Model file for the job. Use its own axes, mm. Face numbers are marked on the shaded views. A direction names the side the tool comes from. Coordinates: 2 decimals unless noted, no trailing zeros. Write each loop counter-clockwise with the first axis right and the second up, starting at its lowest first coordinate (ties: lowest second). Pieces come first, ordered by that corner, then holes. Notation, with made-up numbers: (47.5, 43.5) - (84.5, 43.5) arc R32 ccw to (84.5, 76.5) - close; hole circle Ø4 at (-9, -9.5). An arc over 180 degrees is marked (long way). Put each result on its own line as item: value. Start each with the question number.
1. Saw through at B-B, the plane z = -11. Write the cut outline in (x, y), plus the area to 3 significant figures.
2. Saw through at C-C, the plane x = -28. Write the cut outline in (y, z), plus the area to 3 significant figures.
3. Saw through at A-A, the plane y = -27.5. Write the cut outline in (x, z), plus the area to 3 significant figures.
4. Drop flat-ended pins along their axis: P1, Ø1.5, axis at x = -38, y = -27, coming from the -Z side; P2, Ø1, axis at x = -34, z = 12, coming from the -Y side; P3, Ø3, axis at x = -24, z = 1.5, coming from the +Y side; P4, Ø1.5, axis at x = -39.5, y = -28, coming from the +Z side. Give the stop position or say it passes through.
5. Pull direction Z, two halves, no side cores. Call the marked faces 1, 2, 3 and 4: released by +Z, released by -Z, zero draft, split by the parting line, or undercut.
6. Which spindle directions (+Z, -Z, +X, -X, +Y, -Y) get a long thin tool onto all of the face, cutting with end or side? Do the marked faces 5, 6 and 7. Say none if no direction does.
7. Saw through at D-D, the plane y = -9.75. Write the cut outline in (x, z), plus the area to 3 significant figures.
8. Drill centre lines: L1, parallel to Z at x = -40, y = -27.5; L2, parallel to Z at x = -36, y = -12.5; L3, parallel to Y at x = -34, z = -6. Where is each one in solid material? Low to high. Write a range as from..to.
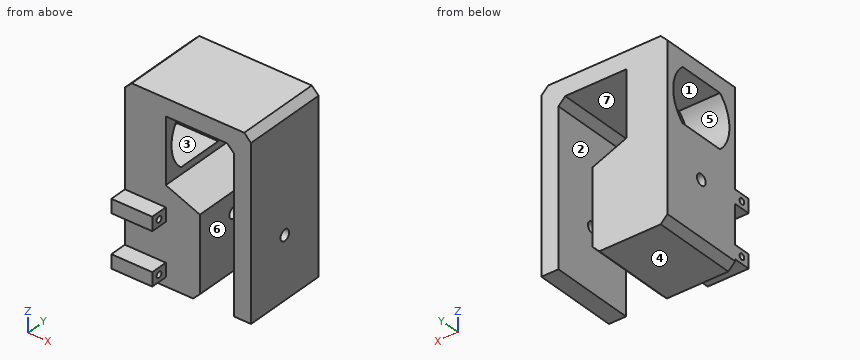
```python
from build123d import *

# Parameters (mm, degrees)
F1_DEPTH = 25
F3_DEPTH = 25
F4_R     = 1.6
F5_DEPTH = 37.001
F6_SIZE  = 2
F7_W     = 5
F7_H     = 4
F7_R     = 0.875
F8_DEPTH = 12


with BuildPart() as f1:
    # F0 (on Front) → F1 (new body)
    with BuildSketch(Plane.XZ):
        Polygon((-8.225309, 26.877944), (-45.225309, 26.877944), (-45.225309, -25.122056), (-23.225309, -25.122056), (-23.225309, -1.122056), (-33.225309, 2.877944), (-33.225309, 21.877944), (-13.225309, 21.877944), (-13.225309, -25.122056), (-8.225309, -25.122056), align=None)
    extrude(amount=F1_DEPTH)

    # F2 (on face) → F3 (cut)
    with BuildSketch(Plane(origin=(-45.225309, 0, 0), x_dir=(0, -1, 0), z_dir=(-1, 0, 0))):
        with BuildLine():
            Line((19.4, 20.441103), (5.6, 20.441103))
            ThreePointArc((5.6, 20.441103), (2.1, 12.659715), (5.6, 4.878327))
            Line((5.6, 4.878327), (19.4, 4.878327))
            ThreePointArc((19.4, 4.878327), (22.9, 12.659715), (19.4, 20.441103))
        make_face()
    extrude(amount=-F3_DEPTH, mode=Mode.SUBTRACT)

    # F4 (on face) → F5 (cut, through all)
    with BuildSketch(Plane(origin=(-45.225309, 0, 0), x_dir=(0, -1, 0), z_dir=(-1, 0, 0))):
        with Locations((12.5, -7.121673)):
            Circle(F4_R)
    extrude(amount=-F5_DEPTH, mode=Mode.SUBTRACT)

    # F6
    f6_edges = [f1.edges().sort_by_distance(p)[0] for p in [
        (-45.225309, -12.5, -25.122056),
        (-23.225309, -12.5, -25.122056),
        (-13.225309, -12.5, 21.877944),
        (-8.225309, -12.5, 26.877944),
        (-45.225309, -12.5, 26.877944),
    ]]
    chamfer(f6_edges, length=F6_SIZE)

    # F7 (on face) → F8 (join, through all)
    with BuildSketch(Plane(origin=(-45.225309, 0, 0), x_dir=(0, -1, 0), z_dir=(-1, 0, 0))):
        with Locations((27.5, -20.542917)):
            Rectangle(F7_W, F7_H)
        with Locations((27.5, -20.542917)):
            Circle(F7_R, mode=Mode.SUBTRACT)
        with Locations((27.5, -5.242917)):
            Rectangle(F7_W, F7_H)
        with Locations((27.5, -5.242917)):
            Circle(F7_R, mode=Mode.SUBTRACT)
    extrude(amount=-F8_DEPTH)


solid = f1.part
```
Final values:
1. outline: (-45.23, -25) - (-23.23, -25) - (-23.23, 0) - (-45.23, 0) - close; (-13.23, -25) - (-8.23, -25) - (-8.23, 0) - (-13.23, 0) - close
1. area: 675 mm²
2. outline: (-25, -25.12) - (0, -25.12) - (0, 0.79) - (-25, 0.79) - close; (-25, 21.88) - (0, 21.88) - (0, 26.88) - (-25, 26.88) - close; hole circle Ø3.2 at (-12.5, -7.12)
2. area: 765 mm²
3. outline: (-45.23, -22.54) - (-33.23, -22.54) - (-33.23, -21.42) - (-45.23, -21.42) - close; (-45.23, -19.67) - (-33.23, -19.67) - (-33.23, -18.54) - (-45.23, -18.54) - close; (-45.23, -7.24) - (-33.23, -7.24) - (-33.23, -6.12) - (-45.23, -6.12) - close; (-45.23, -4.37) - (-33.23, -4.37) - (-33.23, -3.24) - (-45.23, -3.24) - close
3. area: 54.0 mm²
4. P1: stops at z = -22.54
4. P2: stops at y = -25
4. P3: passes through
4. P4: stops at z = -3.24
5. face 1: undercut
5. face 2: zero draft
5. face 3: undercut
5. face 4: released by -Z
6. face 5: -X
6. face 6: -Z, +Y, -Y
6. face 7: +Y, -Y
7. outline: (-45.23, -23.12) - (-43.23, -25.12) - (-25.23, -25.12) - (-23.23, -23.12) - (-23.23, -1.12) - (-33.23, 2.88) - (-33.23, 4.88) - (-45.23, 4.88) - close; (-45.23, 20.44) - (-33.23, 20.44) - (-33.23, 21.88) - (-15.23, 21.88) - (-13.23, 19.88) - (-13.23, -25.12) - (-8.23, -25.12) - (-8.23, 24.88) - (-10.23, 26.88) - (-43.23, 26.88) - (-45.23, 24.88) - close
7. area: 1,050 mm²
8. L1: z = -22.54..-21.42, -19.67..-18.54, -7.24..-6.12, -4.37..-3.24
8. L2: z = -25.12..-8.72, -5.52..4.88, 20.44..26.88
8. L3: y = -30..-27.94, -27.06..-13.64, -11.36..0
